Work out the finished part from the listing and answer in its coordinate system (mm). Face numbers are marked on the shaded views. A direction names the side the tool comes from. Give positions to 0.01 mm unless a question says otherwise; leave off trailing zeros. Loops run counter-clockwise (first coordinate to the right, second up) from the corner with the lowest first, then second, coordinate; pieces in that order, holes last. Notation, with made-up numbers: (89.25, -33.75) - (101.25, -33.75) arc R9 cw to (101.25, -21.75) - close; hole circle Ø7 at (67, -38.5). An arc over 180 degrees is marked (long way). One line per question, with ' | ' between items. Start each with the question number.
1. Section A-A (z = 0) is taken. Determine the outline of the cut face in (x, y), plus the area to 3 significant figures.
2. Section C-C (y = 2.75) is taken. Determine the outline of the cut face in (x, z).
3. Section B-B (x = -1.05) is taken. Determine the outline of the cut face in (y, z).
4. Which of the six approach directions +Z, -Z, +X, -X, +Y, -Y give full straight-line access (tool end or side, diameter ignored) to the marked faces 1, 2, 3 and 4?
5. Section D-D (x = 0) is taken. Determine the outline of the cut face in (y, z), plus the area to 3 significant figures.
6. Find the intervals of material crossed by line 1 (Y direction, x = 0.25, z = 1.3); line 2 (Z direction, x = 0.1, y = 2.5); line 3 (Y direction, x = -1.2, z = -0.55), in increasing order.
7. Each of these flat-tipped pins is pushed along its axis until it touches: pin 1 (1 mm diameter, centred on x = -0.5, z = 1, fed in from -Y); pin 2 (1 mm diameter, centred on x = 0.5, y = -1, fed in from +Z). Where does it stop, or does it pass through?
from build123d import *

# Parameters (mm, degrees)
CROQUIS1_R              = 1.45
SALIENTE_EXTRUIR1_DEPTH = 10.7
CORTAR_EXTRUIR1_START   = -6
CORTAR_EXTRUIR1_DEPTH   = 6
CROQUIS3_R              = 0.5
SALIENTE_EXTRUIR2_DEPTH = 6.4
CUT_EXTRUDE1_START      = -10
CUT_EXTRUDE1_DEPTH      = 10
SKETCH2_W               = 6.740875304
SKETCH2_H               = 8.89846687
CUT_EXTRUDE2_DEPTH      = 11.990677868


with BuildPart() as part:
    # Croquis1 → Saliente-Extruir1 (new body)
    with BuildSketch(Plane(origin=(0, 0, 0), x_dir=(1, 0, 0), z_dir=(0, 1, 0))):
        with Locations(Location((0, 0, 0), (0, 0, 270))):
            Circle(CROQUIS1_R)
    extrude(amount=SALIENTE_EXTRUIR1_DEPTH)

    # Croquis2 → Cortar-Extruir1 (cut)
    with BuildSketch(Plane(origin=(0, 10.7, 0), x_dir=(1, 0, 0), z_dir=(0, 1, 0)).offset(CORTAR_EXTRUIR1_START)):
        with BuildLine():
            Line((-1, -1.05), (1, -1.05))
            ThreePointArc((1, -1.05), (0, -1.45), (-1, -1.05))
        make_face()
    extrude(amount=CORTAR_EXTRUIR1_DEPTH, mode=Mode.SUBTRACT)

    # Croquis3 → Saliente-Extruir2 (add)
    with BuildSketch(Plane.XZ):
        with Locations(Location((0, 0, 0), (0, 0, 270))):
            Circle(CROQUIS3_R)
    extrude(amount=SALIENTE_EXTRUIR2_DEPTH)

    # Sketch1 → Cut-Extrude1 (cut)
    with BuildSketch(Plane(origin=(0, 10.7, 0), x_dir=(1, 0, 0), z_dir=(0, 1, 0)).offset(CUT_EXTRUDE1_START)):
        with BuildLine():
            Line((-1.942782437, 0.6), (1.942782437, 0.6))
            ThreePointArc((1.942782437, 0.6), (0, 2.033323289), (-1.942782437, 0.6))
        make_face()
        with BuildLine():
            Line((-1.942782437, -0.6), (1.942782437, -0.6))
            ThreePointArc((1.942782437, -0.6), (0, -2.033323289), (-1.942782437, -0.6))
        make_face()
    extrude(amount=CUT_EXTRUDE1_DEPTH, mode=Mode.SUBTRACT)

    # Sketch2 → Cut-Extrude2 (cut, through all)
    with BuildSketch(Plane.XY.offset(0.6)):
        with Locations((0.223130537, 7.649233435)):
            Rectangle(SKETCH2_W, SKETCH2_H)
    extrude(amount=-CUT_EXTRUDE2_DEPTH, mode=Mode.SUBTRACT)


solid = part.part
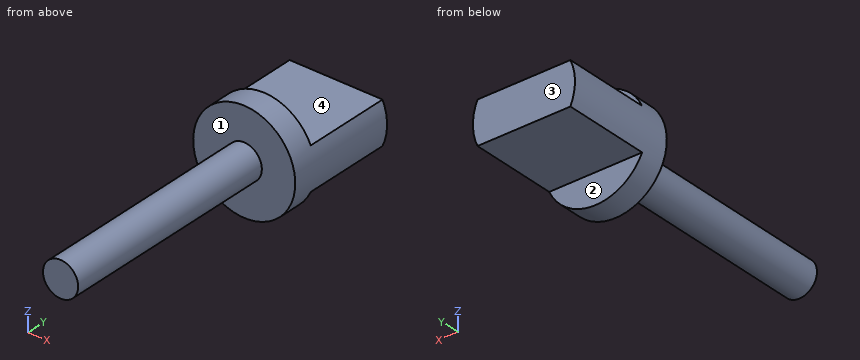
Conclusion:
1) outline: (-1.45, 0) - (-0.5, 0) - (-0.5, -6.4) - (0.5, -6.4) - (0.5, 0) - (1.45, 0) - (1.45, 3.2) - (-1.45, 3.2) - close | area: 15.7 mm²
2) outline: (-1.32, -0.6) - (1.32, -0.6) arc R1.45 ccw to (1.32, 0.6) - (-1.32, 0.6) arc R1.45 ccw to start
3) outline: (0, -1) - (0.7, -1) - (0.7, -0.6) - (3.2, -0.6) - (3.2, 0.6) - (0.7, 0.6) - (0.7, 1) - (0, 1) - close
4) face 1: -Y | face 2: -Z, +X, -X, +Y | face 3: +Z, -Z, +X, -X, +Y | face 4: +Z, +X, -X, +Y
5) outline: (-6.4, -0.5) - (0, -0.5) - (0, -1.45) - (0.7, -1.45) - (0.7, -0.6) - (3.2, -0.6) - (3.2, 0.6) - (0.7, 0.6) - (0.7, 1.45) - (0, 1.45) - (0, 0.5) - (-6.4, 0.5) - close | area: 11.4 mm²
6) line 1: 0 to 0.7 | line 2: -0.6 to 0.6 | line 3: 0 to 3.2
7) pin 1: y = 0 | pin 2: z = 0.5
